Work out the finished part from the listing and answer in its coordinate system (mm). A direction names the side the tool comes from. Give positions to 0.01 mm unless a question says otherwise; leave off trailing zeros. Order: outer loops, then holes, each group sorted by start corner. A loop starts at its lowest first (then second) coordinate and runs counter-clockwise, first axis right, second up. Notation, with made-up numbers: M 2,21 L 6,21 A19 cw 6,32 Z; hole C -37.75,68.25 d11. An arc over 180 degrees is marked long. One line per item, written item: value.
from build123d import *

# Parameters (mm, degrees)
F1_DEPTH = 65.69
F2_W     = 48.438
F2_H     = 131.38
F3_DEPTH = 12.26
F5_DEPTH = 5


# Not quite as in the source:
# - a feature names something its author has since deleted; it is built from what else it names


with BuildPart() as f1:
    # F0 (on Front) → F1 (new body, symmetric)
    with BuildSketch(Plane.XZ):
        with BuildLine():
            Line((-320.0353384018, 0), (-237.2032226722, -27.8760867547))
            Line((-237.2032226722, -27.8760867547), (-188.7652226722, -27.8760867547))
            ThreePointArc((-188.7652226722, -27.8760867547), (-135.7652226722, 33.6790422812), (-82.7652226722, -27.8760867547))
            Line((-82.7652226722, -27.8760867547), (-34.3272226722, -27.8760867547))
            ThreePointArc((-34.3272226722, -27.8760867547), (18.6727773278, 33.6324801702), (71.6727773278, -27.8760867547))
            Line((71.6727773278, -27.8760867547), (120.1107773278, -27.8760867547))
            ThreePointArc((120.1107773278, -27.8760867547), (173.1107773278, 33.6925448374), (226.1107773278, -27.8760867547))
            Line((226.1107773278, -27.8760867547), (274.5487773278, -27.8760867547))
            Line((274.5487773278, -27.8760867547), (357.3808930574, 0))
            Line((357.3808930574, 0), (357.3808930574, 29.795))
            ThreePointArc((357.3808930574, 29.795), (18.6727773278, 60.3473106454), (-320.0353384018, 29.795))
            Line((-320.0353384018, 29.795), (-320.0353384018, 0))
        make_face()
    extrude(amount=F1_DEPTH, both=True)

    # F2 (on face) → F3 (join)
    with BuildSketch(Plane(origin=(0, 0, -27.8760867547), x_dir=(1, 0, 0), z_dir=(0, 0, -1))):
        with BuildLine():
            ThreePointArc((-237.2286491756, -65.5376471925), (-213.0855863574, -89.7567669916), (-188.7906491756, -65.69))
            Line((-188.7906491756, -65.69), (-188.7906491756, 65.8423528075))
            ThreePointArc((-188.7906491756, 65.8423528075), (-212.8485010036, 90.3820549045), (-237.2286491756, 66.1625258279))
            Line((-237.2286491756, 66.1625258279), (-237.2286491756, -65.5376471925))
        make_face()
        with Locations((-58.5462226722, 0)):
            Rectangle(F2_W, F2_H)
        with BuildLine():
            Line((71.6727773278, 65.8423528075), (71.6727773278, -65.69))
            ThreePointArc((71.6727773278, -65.69), (95.8917773278, -89.909), (120.1107773278, -65.69))
            Line((120.1107773278, -65.69), (120.1107773278, 65.8423528075))
            ThreePointArc((120.1107773278, 65.8423528075), (95.8917773278, 90.0613528075), (71.6727773278, 65.8423528075))
        make_face()
        with BuildLine():
            Line((226.1107773278, 65.8423528075), (226.1107773278, -65.69))
            ThreePointArc((226.1107773278, -65.69), (250.3297773278, -89.909), (274.5487773278, -65.69))
            Line((274.5487773278, -65.69), (274.5487773278, 65.8423528075))
            ThreePointArc((274.5487773278, 65.8423528075), (250.3297773278, 90.0613528075), (226.1107773278, 65.8423528075))
        make_face()
        with BuildLine():
            Line((-34.3272226722, -65.69), (-82.7652226722, -65.69))
            ThreePointArc((-82.7652226722, -65.69), (-58.5462226722, -89.909), (-34.3272226722, -65.69))
        make_face()
        with BuildLine():
            ThreePointArc((-34.3272226722, 65.69), (-58.5462226722, 89.909), (-82.7652226722, 65.69))
            Line((-82.7652226722, 65.69), (-34.3272226722, 65.69))
        make_face()
    extrude(amount=F3_DEPTH)

    # F4 (on face) → F5 (join)
    with BuildSketch(Plane.XZ.offset(65.69)):
        with BuildLine():
            ThreePointArc((78.6827773278, -27.8760867547), (18.6727773278, 40.5462292936), (-41.3372226722, -27.8760867547))
            Line((-41.3372226722, -27.8760867547), (-34.3272226722, -27.8760867547))
            ThreePointArc((-34.3272226722, -27.8760867547), (18.6727773278, 33.6324801702), (71.6727773278, -27.8760867547))
            Line((71.6727773278, -27.8760867547), (78.6827773278, -27.8760867547))
        make_face()
        with BuildLine():
            ThreePointArc((233.1207773278, -27.8760867547), (173.1107773278, 40.5405201313), (113.1007773278, -27.8760867547))
            Line((113.1007773278, -27.8760867547), (120.1107773278, -27.8760867547))
            ThreePointArc((120.1107773278, -27.8760867547), (173.1107773278, 33.6925448374), (226.1107773278, -27.8760867547))
            Line((226.1107773278, -27.8760867547), (233.1207773278, -27.8760867547))
        make_face()
        with BuildLine():
            ThreePointArc((-188.7652226722, -27.8760867547), (-135.7652226722, 33.7954088447), (-82.7652226722, -27.8760867547))
            Line((-82.7652226722, -27.8760867547), (-75.7552226722, -27.8760867547))
            ThreePointArc((-75.7552226722, -27.8760867547), (-135.7652226722, 40.6185747484), (-195.7752226722, -27.8760867547))
            Line((-195.7752226722, -27.8760867547), (-188.7906491756, -27.8760867547))
            Line((-188.7906491756, -27.8760867547), (-188.7652226722, -27.8760867547))
        make_face()
    extrude(amount=F5_DEPTH)

    # F6: F1 across plane


with BuildPart() as f1_1:
    add(f1.part)
    add(f1.part.mirror(Plane.XZ))


solid = f1_1.part
(1) Section C-C, the plane z = 11 is taken. Give the number of separate pieces and of enclosed holes in the cut face, then the cut area to 3 significant figures.
Findings:
separate pieces: 4
enclosed holes: 0
area: 55,000 mm^2
(2) Section B-B, the plane x = -147 is taken. Give the vertices of the cut face in (y, z).
Findings:
outline: M -70.69,32.6 L -65.69,32.6 L -65.69,32.49 L 65.69,32.49 L 65.69,32.6 L 70.69,32.6 L 70.69,39.57 L 65.69,39.57 L 65.69,53.08 L -65.69,53.08 L -65.69,39.57 L -70.69,39.57 Z
(3) Section D-D, the plane x = 141.5 is taken. Give the vertices of the cut face in (y, z), then the cut area to 3 significant figures.
Findings:
outline: M -70.69,23.38 L 70.69,23.38 L 70.69,31.63 L 65.69,31.63 L 65.69,56.36 L -65.69,56.36 L -65.69,31.63 L -70.69,31.63 Z
area: 4,420 mm^2
(4) Given P1, Ø1.5, axis at x = 208.5, z = 21, coming from the -Y side; P2, Ø4, axis at x = -43, z = 31.5, coming from the -Y side; P3, Ø3, axis at x = 200, y = 32, coming from the +Z side, each flat-ended and moving along its own axis, determine where each tip first touches the part or whether it passes through.
Findings:
P1: stops at y = -70.69
P2: stops at y = -65.69
P3: stops at z = 51.79
(5) Determine the mould class of faces 5 (the flat face through (-237.229, -1, -34)), 6 (the flat face through (96, 1, -40.136)), 7 (the cylindrical face through (250.862, -90.055, -33.92)) for opening direction X: pulls with the +X half, pulls with the -X half, needs draft (parallel to the pull), parting line crosses it, or undercut.
Findings:
face 5: pulls with the -X half
face 6: needs draft
face 7: undercut
(6) Which of the six approach directions +Z, -Z, +X, -X, +Y, -Y give full straight-line access (tool end or side, diameter ignored) to faces 1 (the flat face through (173, 70.69, 34)), 2 (the flat face through (14, -70.69, 34)), 3 (the flat face through (71.673, 1, -34)), 4 (the flat face through (357.381, -1, 15))?
Findings:
face 1: +Z, +X, -X, +Y
face 2: +Z, +X, -X, -Y
face 3: -Z, +Y, -Y
face 4: +Z, -Z, +X, +Y, -Y
(7) Find the intervals of material crossed by probe 1 along X at (y, z) = (-1.5, 21.5); probe 2 along X at (y, z) = (-61, 25); probe 3 along Y at (x, z) = (-277, 25.5), in increasing order. Write a range as from..to.
Findings:
probe 1: x = -320.04..-169.78, -101.75..-15.28, 52.63..139.08, 207.14..357.38
probe 2: x = -320.04..-165.01, -106.53..-10.49, 47.84..143.85, 202.37..357.38
probe 3: y = -65.69..65.69
